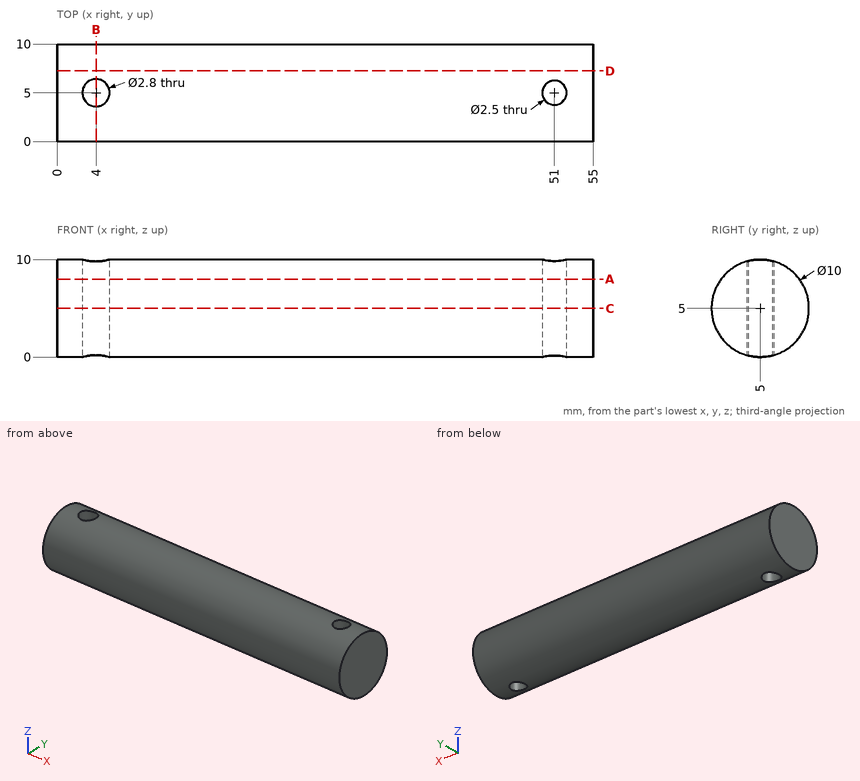
The figure shows three views and two pictorial views of one solid part (mm, origin at its lowest corner). Answer the questions. Round coordinates to 2 decimals unless told otherwise and drop trailing zeros. Write each loop counter-clockwise with the first axis right and the second up, starting at its lowest first coordinate (ties: lowest second). Pieces come first, ordered by that corner, then holes. Notation, with made-up numbers: (11.25, 25.5) -> (47.25, 25.5) arc R22 ccw to (47.25, 43.5) -> close; hole circle Ø10 at (7.25, -3.5). An arc over 180 degrees is marked (long way). Answer as a JSON object with one key per item and string values. Group by question number.
Q1. Section C-C (z = 5) is taken. Write down the section's boundary in (x, y).
Q2. Section D-D (y = 7.25) is taken. Write down the section's boundary in (x, z).
Q3. Straight lines are drawn through the part: line 1 along X through (y, z) = (6, 1.75); line 2 along Y through (x, z) = (51, 4.75); line 3 along Y through (x, z) = (4, 5.5). For each, find the intervals that lie inside material, in ascending order.
Q4. Section A-A (z = 8) is taken. Write down the section's boundary in (x, y).
Q5. Section B-B (x = 4) is taken. Write down the section's boundary in (y, z), plus the area to 3 significant figures.
Q6. Each of these flat-tipped pins is pushed along its axis until it touches: pin 1 Ø6 at (x, y) = (8.5, 8.5) entering from -Z; pin 2 Ø4 at (x, z) = (40.5, 6.5) entering from +Y; pin 3 Ø1 at (x, y) = (35.5, 3.5) entering from -Z; pin 4 Ø3 at (x, z) = (48, 8.5) entering from -Y. Where does it stop, or does it pass through?
Check values:
{
 "1": {"outline": "(0, 0) -> (55, 0) -> (55, 10) -> (0, 10) -> close; hole circle Ø2.8 at (4, 5); hole circle Ø2.5 at (51, 5)"},
 "2": {"outline": "(0, 0.53) -> (55, 0.53) -> (55, 9.47) -> (0, 9.47) -> close"},
 "3": {"line 1": "0 to 3.02, 4.98 to 50.25, 51.75 to 55", "line 2": "0.01 to 3.75, 6.25 to 9.99", "line 3": "0.03 to 3.6, 6.4 to 9.97"},
 "4": {"outline": "(0, 1) -> (55, 1) -> (55, 9) -> (0, 9) -> close; hole circle Ø2.8 at (4, 5); hole circle Ø2.5 at (51, 5)"},
 "5": {"outline": "(3.6, 0.2) -> (3.6, 9.8) arc R5 ccw to start; (6.4, 0.2) arc R5 ccw to (6.4, 9.8) -> close", "area": "50.9 mm^2"},
 "6": {"pin 1": "z = 0.03", "pin 2": "y = 10", "pin 3": "z = 0.1", "pin 4": "y = 0.42"}
}
